The listing builds one solid part. Answer for the finished solid, in the listing's coordinates (mm). A direction names the side the tool comes from. Round coordinates to 2 decimals unless told otherwise and drop trailing zeros. Write each loop counter-clockwise with the first axis right and the second up, starting at its lowest first coordinate (ties: lowest second). Pieces come first, ordered by that corner, then holes.
Item 1: Find section D-D on y = 5.5. Give the vertices of the cut face in (x, z).
Item 2: Each of these flat-tipped pins is pushed along its axis until it touches: pin 1 (3 mm diameter, centred on x = -5.5, y = 0, fed in from -Z); pin 2 (1 mm diameter, centred on y = 2.5, z = 1.5, fed in from -X); pin 3 (1 mm diameter, centred on x = -20, z = 1, fed in from +Y). Where does it stop, or does it pass through?
Item 3: Find section A-A on y = 0. Give the vertices of the cut face in (x, z) (3 decimals), then the cut area to 3 significant figures.
Item 4: Find section B-B on x = -27. Give the vertices of the cut face in (y, z).
Item 5: For a pull along Y with two mould halves and no side action, classify faces 5 (the face through (-17, -2, 2)), 6 (the face through (-51.056, -1.159, 0.986)), 7 (the face through (-57.85, -0.09, 0.99)) as +Y half, -Y half, draft (parallel to the pull), parting line (faces both ways), or undercut.
Item 6: Find the intervals of material crossed by probe 1 along Y at (x, z) = (0, 0.95) (3 decimals); probe 2 along Y at (x, z) = (-38, 0.1); probe 3 along X at (y, z) = (-2, 0.3), in increasing order.
Item 7: Find section C-C on z = 1.2. Give the vertices of the cut face in (x, y) (3 decimals), then the cut area to 3 significant figures.
Item 8: A tool of negligible diameter and unlimited length cuts with its end or side. For faces 1 (the face through (-30, 4, 1)), 2 (the face through (-17, -2, 0)), 3 (the face through (-29, -1.483, 1)), 4 (the face through (-30, -4, 1)), from which of +Z, -Z, +X, -X, +Y, -Y can it reach the whole face along a straight path? Write none if from no direction.
```python
from build123d import *

# Parameters (mm, degrees)
SKETCH_1_R          = 1
SKETCH_1_R_2        = 3.025
SKETCH_1_R_3        = 1.5
EXTRUDE_1_DEPTH     = 2
SKETCH_2_R          = 3.025
CUT_EXTRUDE_1_DEPTH = 10


with BuildPart() as part:
    # 草图1 → 凸台-拉伸1 (new body)
    with BuildSketch(Plane.XY):
        with BuildLine():
            Line((-53.850242828, 4), (-6.34428877, 4))
            ThreePointArc((-6.34428877, 4), (7.5, 0), (-6.34428877, -4))
            Line((-6.34428877, -4), (-53.850242828, -4))
            ThreePointArc((-53.850242828, -4), (-57.850242828, 0), (-53.850242828, 4))
        make_face()
        with Locations((0, 5.5)):
            Circle(SKETCH_1_R, mode=Mode.SUBTRACT)
        with Locations((0, -5.5)):
            Circle(SKETCH_1_R, mode=Mode.SUBTRACT)
        with Locations((-53.850242828, 0)):
            Circle(SKETCH_1_R_2, mode=Mode.SUBTRACT)
        Circle(SKETCH_1_R_3, mode=Mode.SUBTRACT)
        with Locations((-5.5, 0)):
            Circle(SKETCH_1_R, mode=Mode.SUBTRACT)
        with Locations((5.5, 0)):
            Circle(SKETCH_1_R, mode=Mode.SUBTRACT)
        with BuildLine():
            ThreePointArc((-10.194558278, -1.483471582), (-8.711086696, 0), (-10.194558278, 1.483471582))
            Line((-10.194558278, 1.483471582), (-47.761926325, 1.483471582))
            ThreePointArc((-47.761926325, 1.483471582), (-49.245397907, 0), (-47.761926325, -1.483471582))
            Line((-47.761926325, -1.483471582), (-10.194558278, -1.483471582))
        make_face(mode=Mode.SUBTRACT)
    extrude(amount=EXTRUDE_1_DEPTH)

    # 草图2 → 切除-拉伸1 (cut)
    with BuildSketch(Plane.XY.offset(2)):
        Circle(SKETCH_2_R)
    extrude(amount=-CUT_EXTRUDE_1_DEPTH, mode=Mode.SUBTRACT)


solid = part.part
```
Check values:
1. outline: (-5.1, 0) - (-1, 0) - (-1, 2) - (-5.1, 2) - close; (1, 0) - (5.1, 0) - (5.1, 2) - (1, 2) - close
2. pin 1: stops at z = 0
2. pin 2: stops at x = -57.31
2. pin 3: stops at y = 4
3. outline: (-57.85, 0) - (-56.875, 0) - (-56.875, 2) - (-57.85, 2) - close; (-50.825, 0) - (-49.245, 0) - (-49.245, 2) - (-50.825, 2) - close; (-8.711, 0) - (-6.5, 0) - (-6.5, 2) - (-8.711, 2) - close; (-4.5, 0) - (-3.025, 0) - (-3.025, 2) - (-4.5, 2) - close; (3.025, 0) - (4.5, 0) - (4.5, 2) - (3.025, 2) - close; (6.5, 0) - (7.5, 0) - (7.5, 2) - (6.5, 2) - close
3. area: 17.4 mm2
4. outline: (-4, 0) - (-1.48, 0) - (-1.48, 2) - (-4, 2) - close; (1.48, 0) - (4, 0) - (4, 2) - (1.48, 2) - close
5. face 5: draft
5. face 6: undercut
5. face 7: parting line
6. probe 1: y = -7.5 to -6.5, -4.5 to -3.025, 3.025 to 4.5, 6.5 to 7.5
6. probe 2: y = -4 to -1.48, 1.48 to 4
6. probe 3: x = -57.31 to -56.12, -51.58 to -2.27, 2.27 to 7.23
7. outline: (-53.85, -4) - (-6.344, -4) arc R7.5 ccw (long way) to (-6.344, 4) - (-53.85, 4) arc R4 ccw to start; hole circle Ø6.05 at (-53.85, 0); hole (-47.762, -1.483) - (-10.195, -1.483) arc R1.483 ccw to (-10.195, 1.483) - (-47.762, 1.483) arc R1.483 ccw to start; hole circle Ø2 at (-5.5, 0); hole circle Ø6.05 at (0, 0); hole circle Ø2 at (0, -5.5); hole circle Ø2 at (0, 5.5); hole circle Ø2 at (5.5, 0)
7. area: 387 mm2
8. face 1: +Z, -Z, -X, +Y
8. face 2: -Z, +X, -X, +Y, -Y
8. face 3: +Z, -Z
8. face 4: +Z, -Z, -X, -Y
